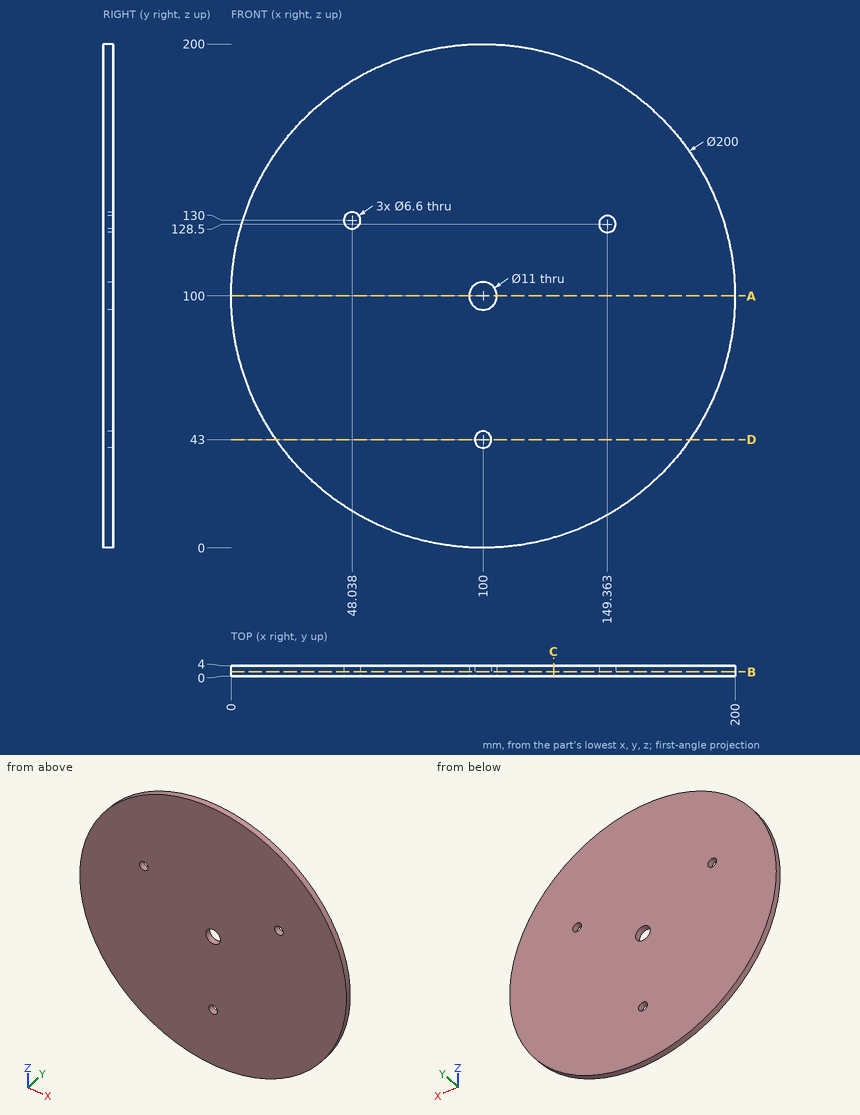
Geometry: see drawing. Coordinates: mm, zero at the bounding-box minimum. Coordinates: 2 decimals unless noted, no trailing zeros. Order: outer loops, then holes, each group sorted by start corner. A loop starts at its lowest first (then second) coordinate and runs counter-clockwise, first axis right, second up. Notation, with made-up numbers: M 43.25,35.5 L 69.25,35.5 A24 cw 69.25,54.5 Z; hole C 5,74.25 d5. An arc over 180 degrees is marked long. Write item = value, one per line. Start each with the question number.
(1) Line query: line 1 along Z through (x, y) = (100, 2.5); line 2 along X through (y, z) = (1.25, 130) (1 decimal); line 3 along X through (y, z) = (0.95, 128.5) (1 decimal). Output: solid intervals per line, ascending. Write a range as [from, to].
(2) Section D-D on z = 43. Output: boundary loops of the cut face in (x, y) (1 decimal).
(3) First-contact query: P1, Ø1, axis at y = 2, z = 71, coming from the +X side; P2, Ø2, axis at y = 2, z = 53.5, coming from the -X side; P3, Ø1, axis at y = 2.5, z = 165.5, coming from the +X side (1 decimal); P4, Ø10, axis at x = 100, z = 100, coming from the +Y side. Flat tips, straight axial feed; report the tip coordinate or a pass-through.
(4) Section B-B on y = 1.65. Output: boundary loops of the cut face in (x, z), and give its area (3 significant figures).
(5) Section A-A on z = 100. Output: boundary loops of the cut face in (x, y), and give its area (3 significant figures).
(6) Section C-C on x = 128. Output: boundary loops of the cut face in (y, z).
Result set:
q1.line_1 = [0, 39.7], [46.3, 94.5], [105.5, 200]
q1.line_2 = [4.6, 44.7], [51.3, 146.4], [152.3, 195.4]
q1.line_3 = [4.1, 45.1], [51, 146.1], [152.7, 195.9]
q2.outline = M 17.8,0 L 96.7,0 L 96.7,4 L 17.8,4 Z; M 103.3,0 L 182.2,0 L 182.2,4 L 103.3,4 Z
q3.P1 = 195.85
q3.P2 = 10.95
q3.P3 = 176
q3.P4 = through
q4.outline = C 100,100 d200; hole C 48.04,130 d6.6; hole C 100,100 d11; hole C 100,43 d6.6; hole C 149.36,128.5 d6.6
q4.area = 31,200 mm²
q5.outline = M 0,0 L 94.5,0 L 94.5,4 L 0,4 Z; M 105.5,0 L 200,0 L 200,4 L 105.5,4 Z
q5.area = 756 mm²
q6.outline = M 0,4 L 4,4 L 4,196 L 0,196 Z
